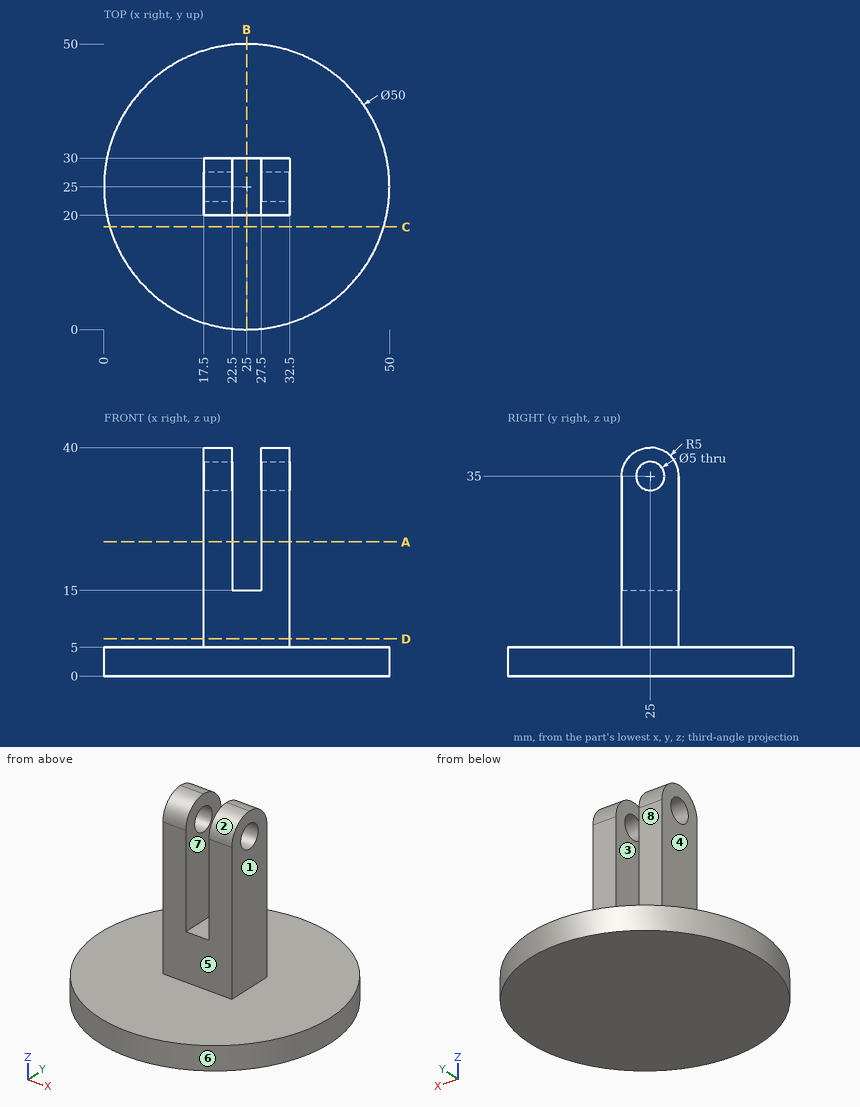
Source: three-view drawing plus pictorial views. Frame: mm from the lowest corner of the part. A direction names the side the tool comes from. Round coordinates to 2 decimals unless told otherwise and drop trailing zeros. Write each loop counter-clockwise with the first axis right and the second up, starting at its lowest first coordinate (ties: lowest second). Pieces come first, ordered by that corner, then holes. Notation, with made-up numbers: M 43.25,32.5 L 62.25,32.5 A12 ccw 62.25,45.5 Z; hole C 1.25,56.25 d7. An arc over 180 degrees is marked long. Use CSV: the item, a comma, the result in double quotes. Start each with the question number.
Q1. Pull-direction query (X, two-part tool) for the marked faces 1, 2 and 3; classes: +X half, -X half, draft (parallel to the pull), parting line (faces both ways), or undercut.
Q2. Cut plane A-A on z = 23.5. Output: boundary loops of the cut face in (x, y), plus the area to 3 significant figures.
Q3. Line query: line 1 (Z direction, x = 31.5, y = 25); line 2 (X direction, y = 29.5, z = 36.5); line 3 (Z direction, x = 40, y = 27). Output: solid intervals per line, ascending. Write a range as from..to.
Q4. Cut plane D-D on z = 6.5. Output: boundary loops of the cut face in (x, y), plus the area to 3 significant figures.
Q5. Cut plane C-C on y = 18. Output: boundary loops of the cut face in (x, z).
Q6. Cut plane B-B on x = 25. Output: boundary loops of the cut face in (y, z).
Q7. Access query for the marked faces 4, 5, 6, 7 and 8. Directions: +Z, -Z, +X, -X, +Y, -Y. A direction counts if a zero-diameter tool reaches every point of the face in a straight line with its end or side. Return the directions, or none.
Q8. First-contact query: P1, Ø11, axis at y = 26, z = 22, coming from the +X side; P2, Ø12, axis at x = 27, z = 22.5, coming from the -Y side; P3, Ø3, axis at y = 24, z = 31, coming from the -X side; P4, Ø1, axis at x = 16.5, z = 19, coming from the +Y side. Flat tips, straight axial feed; report the tip coordinate or a pass-through.
Results found:
1,face 1,"+X half"
1,face 2,"draft"
1,face 3,"undercut"
2,outline,"M 17.5,20 L 22.5,20 L 22.5,30 L 17.5,30 Z; M 27.5,20 L 32.5,20 L 32.5,30 L 27.5,30 Z"
2,area,"100 mm^2"
3,line 1,"0..32.5, 37.5..40"
3,line 2,"17.5..22.5, 27.5..32.5"
3,line 3,"0..5"
4,outline,"M 17.5,20 L 32.5,20 L 32.5,30 L 17.5,30 Z"
4,area,"150 mm^2"
5,outline,"M 1,0 L 49,0 L 49,5 L 1,5 Z"
6,outline,"M 0,0 L 50,0 L 50,5 L 30,5 L 30,15 L 20,15 L 20,5 L 0,5 Z"
7,face 4,"+Z, -X, +Y, -Y"
7,face 5,"+Z, +X, -X, -Y"
7,face 6,"+Z, -Z"
7,face 7,"+Z, +Y, -Y"
7,face 8,"+Z, +X, -X, +Y"
8,P1,"x = 32.5"
8,P2,"y = 20"
8,P3,"x = 17.5"
8,P4,"through"
